Could you check a few things on this model? Use its own coordinates, in mm. A direction names the side the tool comes from. Coordinates: 2 decimals unless noted, no trailing zeros. Loops run counter-clockwise (first coordinate to the right, second up) from the corner with the lowest first, then second, coordinate; pieces in that order, holes last.
from build123d import *

# Parameters (mm, degrees)
F1_DEPTH = 28.575
F2_W     = 44.45
F2_H     = 44.45
F3_DEPTH = 127
F4_R     = 6.35
F5_DEPTH = 57.151


with BuildPart() as f1:
    # F0 (on Front) → F1 (new body, symmetric)
    with BuildSketch(Plane.XZ):
        Polygon((-50.8, 25.4), (-50.8, 0), (50.8, 0), (50.8, 25.4), (44.247393, 50.8), (-43.547828, 50.8), align=None)
    extrude(amount=F1_DEPTH, both=True)

    # F2 (on face) → F3 (cut)
    with BuildSketch(Plane(origin=(-50.8, 0, 0), x_dir=(0, -1, 0), z_dir=(-1, 0, 0))):
        with Locations((0, 28.575)):
            Rectangle(F2_W, F2_H)
    extrude(amount=-F3_DEPTH, mode=Mode.SUBTRACT)

    # F4 (on face) → F5 (cut, through all)
    with BuildSketch(Plane(origin=(0, 28.575, 0), x_dir=(-1, 0, 0), z_dir=(0, 1, 0))):
        with Locations((0, 38.1)):
            Circle(F4_R)
    extrude(amount=-F5_DEPTH, mode=Mode.SUBTRACT)


solid = f1.part
(1) For pin 1 (8 mm diameter, centred on x = -23.5, y = 6, fed in from +Z); pin 2 (16.5 mm diameter, centred on x = 0, z = 38.1, fed in from -Y) (3 decimals), each with a flat end and sliding along its axis, tell me the tip position at first contact or that it passes through.
Answers:
pin 1: stops at z = 6.35
pin 2: stops at y = -28.575
(2) Imagine slicing it at D-D, the plane y = 14.5. Write out the boundary of the cut face in (x, z), and give its area (3 significant figures).
Answers:
outline: (-50.8, 0) - (50.8, 0) - (50.8, 6.35) - (-50.8, 6.35) - close
area: 645 mm2
(3) I need wall thicknesses on probe 1 along Y at (x, z) = (44.5, 28.5) (3 decimals); probe 2 along Z at (x, y) = (-43.5, 9); probe 3 along Z at (x, y) = (0, -25). Which ranges of each line are inside material? Lowest first, please.
Answers:
probe 1: y = -28.575 to -22.225, 22.225 to 28.575
probe 2: z = 0 to 6.35
probe 3: z = 0 to 31.75, 44.45 to 50.8
(4) Imagine slicing it at A-A, the plane x = 0. Write out the boundary of the cut face in (y, z) (3 decimals), and give its area (3 significant figures).
Answers:
outline: (-28.575, 0) - (28.575, 0) - (28.575, 31.75) - (22.225, 31.75) - (22.225, 6.35) - (-22.225, 6.35) - (-22.225, 31.75) - (-28.575, 31.75) - close; (-28.575, 44.45) - (-22.225, 44.45) - (-22.225, 50.8) - (-28.575, 50.8) - close; (22.225, 44.45) - (28.575, 44.45) - (28.575, 50.8) - (22.225, 50.8) - close
area: 766 mm2
(5) Imagine slicing it at B-B, the plane z = 12. Write out the boundary of the cut face in (x, y) (3 decimals).
Answers:
outline: (-50.8, -28.575) - (50.8, -28.575) - (50.8, -22.225) - (-50.8, -22.225) - close; (-50.8, 22.225) - (50.8, 22.225) - (50.8, 28.575) - (-50.8, 28.575) - close
(6) Which directions (+Z, -Z, +X, -X, +Y, -Y) give clear straight access to the entire face, cutting with the end or side of a thin tool? Please do faces 1 (the face through (-1, -28.575, 26)), 2 (the face through (-1, -22.225, 28)).
Answers:
face 1: +Z, -Z, +X, -X, -Y
face 2: +Z, +X, -X
(7) We'd pull the mould along Y, two halves only. Please class faces 3 (the face through (-1, 22.225, 28)), 4 (the face through (-47.123, -25.444, 38.278)), 5 (the face through (-1, 28.575, 26)): +Y half, -Y half, draft (parallel to the pull), parting line (faces both ways), or undercut.
Answers:
face 3: undercut
face 4: draft
face 5: +Y half
(8) Imagine slicing it at C-C, the plane z = 37. Write out the boundary of the cut face in (x, y) (3 decimals), and give its area (3 significant figures).
Answers:
outline: (-47.488, -28.575) - (-6.254, -28.575) - (-6.254, -22.225) - (-47.488, -22.225) - close; (-47.488, 22.225) - (-6.254, 22.225) - (-6.254, 28.575) - (-47.488, 28.575) - close; (6.254, -28.575) - (47.807, -28.575) - (47.807, -22.225) - (6.254, -22.225) - close; (6.254, 22.225) - (47.807, 22.225) - (47.807, 28.575) - (6.254, 28.575) - close
area: 1,050 mm2
